from build123d import *

# Parameters (mm, degrees)
BOSS_EXTRUDE1_DEPTH = 6.35
CIRPATTERN1_COUNT   = 18
SKETCH2_R           = 1.5
CUT_EXTRUDE1_DEPTH  = 6.35


with BuildPart() as part:
    # Sketch1 → Boss-Extrude1 (new body)
    with BuildSketch(Plane(origin=(0, 0, 0), x_dir=(1, 0, 0), z_dir=(0, 1, 0))):
        with BuildLine():
            Line((0, 0), (-1.880045408, 10.66226734))
            ThreePointArc((-1.880045408, 10.66226734), (-1.413174452, 10.734125653), (-0.943613438, 10.785550948))
            Line((-0.943613438, 10.785550948), (-1.029695335, 11.769471531))
            ThreePointArc((-1.029695335, 11.769471531), (-0.972041848, 12.892396814), (-0.609362841, 13.956703655))
            ThreePointArc((-0.609362841, 13.956703655), (0, 13.97), (0.609362841, 13.956703655))
            ThreePointArc((0.609362841, 13.956703655), (0.972041848, 12.892396814), (1.029695335, 11.769471531))
            Line((1.029695335, 11.769471531), (0.943613438, 10.785550948))
            ThreePointArc((0.943613438, 10.785550948), (1.413174452, 10.734125653), (1.880045408, 10.66226734))
            Line((1.880045408, 10.66226734), (0, 0))
        make_face()
    boss_extrude1 = extrude(amount=BOSS_EXTRUDE1_DEPTH)

    # CirPattern1: Boss-Extrude1 ×18 about axis
    cirpattern1_axis = Axis((0, 0, 0), (0, 1, 0))
    for i in range(1, CIRPATTERN1_COUNT):
        add(boss_extrude1.rotate(cirpattern1_axis, i * 360 / CIRPATTERN1_COUNT))

    # Sketch2 → Cut-Extrude1 (cut)
    with BuildSketch(Plane(origin=(0, 6.35, 0), x_dir=(1, 0, 0), z_dir=(0, 1, 0))):
        Circle(SKETCH2_R)
    extrude(amount=-CUT_EXTRUDE1_DEPTH, mode=Mode.SUBTRACT)


solid = part.part
The model under review builds one solid part; all positions refer to its coordinate system, in mm. A direction names the side the tool comes from. Round coordinates to 2 decimals unless told otherwise and drop trailing zeros. Order: outer loops, then holes, each group sorted by start corner. A loop starts at its lowest first (then second) coordinate and runs counter-clockwise, first axis right, second up. Notation, with made-up numbers: (64, 58) -> (73, 58) arc R20 ccw to (73, 74) -> close; hole circle Ø6 at (-30.75, 2.25). An arc over 180 degrees is marked (long way). Return JSON: item names as keys, results as strings.
1. For faces 4 (the face through (5.32, 3.13, 11.77)), 5 (the face through (4.786, 3.131, 13.125)), 6 (the face through (2.93, 3.13, -10.93)), 7 (the face through (11.284, 3.131, -0.987)), 8 (the face through (7.555, 3.131, 10.511)), list the 3-axis set-ups (+Z, -Z, +X, -X, +Y, -Y) from which the entire face can be reached by the end or side of a thin tool; tool diameter is ignored.
Answer block:
{"face 4": "+Y, -Y", "face 5": "+Z, +X, +Y, -Y", "face 6": "-Z, +Y, -Y", "face 7": "+X, +Y, -Y", "face 8": "+Z, +Y, -Y"}
2. Take a section at A-A (x = 0). Write out the cut boundary in (y, z).
Answer block:
{"outline": "(0, -13.97) -> (6.35, -13.97) -> (6.35, -1.5) -> (0, -1.5) -> close; (0, 1.5) -> (6.35, 1.5) -> (6.35, 13.97) -> (0, 13.97) -> close"}
3. For L1, parallel to Z at x = -10.5, y = 2.25; L2, parallel to Z at x = 0, y = 1.75; L3, parallel to Z at x = -12, y = 2.25, list the stretches that pass through material, from the lowest coordinate up. Write a range as [from, to].
Answer block:
{"L1": "z = [-7.22, -4.9], [-2.81, 2.81], [4.9, 7.22]", "L2": "z = [-13.97, -1.5], [1.5, 13.97]", "L3": "z = [-7.15, -5.94], [-3.17, -1.06], [1.06, 3.17], [5.94, 7.15]"}
4. The part is to be moulded in two halves that separate along Z. For faces 1 (the face through (-2.93, 3.13, 10.93)), 2 (the face through (0.986, 3.131, 11.271)), 3 (the face through (-0.01, 3.13, -13.97)), say which applies: +Z half, -Z half, draft (parallel to the pull), parting line (faces both ways), or undercut.
Answer block:
{"face 1": "+Z half", "face 2": "undercut", "face 3": "-Z half"}
